The model under review builds one solid part; all positions refer to its coordinate system, in mm. Give positions to 0.01 mm unless a question says otherwise; leave off trailing zeros. Put each result on its own line as item: value.
```python
from build123d import *

# Parameters (mm, degrees)
SKETCH_3_R      = 1.700000006
SKETCH_3_R_2    = 1.100000006
SKETCH_3_W      = 12.5
SKETCH_3_H      = 23.5
EXTRUDE_2_DEPTH = 2


with BuildPart() as part:
    # 草图3 → 凸台-拉伸2 (new body)
    with BuildSketch(Plane.XY):
        with BuildLine():
            Line((16.840804288, 56.117583031), (0.840804288, 56.117583031))
            ThreePointArc((0.840804288, 56.117583031), (-0.573409274, 55.531796593), (-1.159195712, 54.117583031))
            Line((-1.159195712, 54.117583031), (-1.159195712, -100.882416969))
            ThreePointArc((-1.159195712, -100.882416969), (8.840804288, -110.882416969), (18.840804288, -100.882416969))
            Line((18.840804288, -100.882416969), (18.840804288, 54.117583031))
            ThreePointArc((18.840804288, 54.117583031), (18.255017851, 55.531796593), (16.840804288, 56.117583031))
        make_face()
        with Locations((8.840804288, -107.982416969)):
            Circle(SKETCH_3_R, mode=Mode.SUBTRACT)
        with BuildLine():
            ThreePointArc((10.540804288, -93.782416969), (7.63872276, -94.984498497), (8.840804288, -92.082416969))
            ThreePointArc((8.840804288, -92.082416969), (10.042885816, -92.580335441), (10.540804288, -93.782416969))
        make_face(mode=Mode.SUBTRACT)
        with BuildLine():
            ThreePointArc((10.540804294, -46.401557681), (10.04288582, -47.603639213), (8.840804288, -48.101557686))
            ThreePointArc((8.840804288, -48.101557686), (7.638722756, -45.199476149), (10.540804294, -46.401557681))
        make_face(mode=Mode.SUBTRACT)
        with Locations((8.840804288, -39.301557681)):
            Circle(SKETCH_3_R, mode=Mode.SUBTRACT)
        with Locations((8.840804288, -32.201557681)):
            Circle(SKETCH_3_R, mode=Mode.SUBTRACT)
        with Locations((8.840804288, -100.882416969)):
            Circle(SKETCH_3_R, mode=Mode.SUBTRACT)
        with BuildLine():
            add(Edge.make_bspline(
                [(8.840804288, -68.07230608), (10.518584029, -67.9276906), (13.271622127, -65.4378125), (9.324741551, -63.725127446)],
                knots=[0.615915535, 0.615915535, 0.615915535, 0.615915535, 1, 1, 1, 1], degree=3))
            add(Edge.make_bspline(
                [(5.004317127, -62.675716717), (6.671990842, -63.522758583), (7.358746233, -65.159768504), (7.765991833, -67.969605562), (8.568188953, -68.095804038), (8.840804288, -68.07230608)],
                knots=[0.002348501, 0.002348501, 0.002348501, 0.002348501, 0.410926836, 0.553507274, 0.615915535, 0.615915535, 0.615915535, 0.615915535], degree=3))
            add(Edge.make_bspline(
                [(4.975444833, -62.661146677), (4.985052333, -62.666591164), (4.994678321, -62.671455775), (5.004317127, -62.675716717)],
                knots=[0.565822578, 0.565822578, 0.565822578, 0.565822578, 0.579602808, 0.579602808, 0.579602808, 0.579602808], degree=3))
            add(Edge.make_bspline(
                [(4.278018154, -60.704640985), (4.226627162, -61.157219039), (4.526861731, -62.258746315), (4.916709377, -62.627861804), (4.975444833, -62.661146677)],
                knots=[0, 0, 0, 0, 0.481577142, 0.565822578, 0.565822578, 0.565822578, 0.565822578], degree=3))
            add(Edge.make_bspline(
                [(4.278018154, -60.704640985), (4.226627162, -60.252062931), (4.526861731, -59.150535655), (4.916709377, -58.781420166), (4.975444833, -58.748135293)],
                knots=[0, 0, 0, 0, 0.481577142, 0.565822578, 0.565822578, 0.565822578, 0.565822578], degree=3))
            add(Edge.make_bspline(
                [(4.975444833, -58.748135293), (4.985052333, -58.742690806), (4.994678321, -58.737826195), (5.004317127, -58.733565253)],
                knots=[0.565822578, 0.565822578, 0.565822578, 0.565822578, 0.579602808, 0.579602808, 0.579602808, 0.579602808], degree=3))
            add(Edge.make_bspline(
                [(5.004317127, -58.733565253), (6.671990842, -57.886523387), (7.358746233, -56.249513466), (7.765991833, -53.439676408), (8.568188953, -53.313477932), (8.840804288, -53.33697589)],
                knots=[0.002348501, 0.002348501, 0.002348501, 0.002348501, 0.410926836, 0.553507274, 0.615915535, 0.615915535, 0.615915535, 0.615915535], degree=3))
            add(Edge.make_bspline(
                [(8.840804288, -53.33697589), (10.518584029, -53.481591371), (13.271622127, -55.97146947), (9.324741551, -57.684154524)],
                knots=[0.615915535, 0.615915535, 0.615915535, 0.615915535, 1, 1, 1, 1], degree=3))
            add(Edge.make_bspline(
                [(9.324741551, -57.684154524), (9.448361201, -57.741607127), (9.579397012, -57.825403241)],
                knots=[0.879374293, 0.879374293, 0.879374293, 1, 1, 1], degree=2))
            add(Edge.make_bspline(
                [(9.579397012, -57.825403241), (10.442809677, -57.472287252), (11.335132803, -57.233463092), (12.256366661, -57.108930725)],
                knots=[0, 0, 0, 0, 0.985819408, 0.985819408, 0.985819408, 0.985819408], degree=3))
            add(Edge.make_bspline(
                [(12.256366661, -57.108930725), (12.250375457, -57.017628974), (12.324042897, -56.451578095), (14.134987008, -56.284356721), (14.027647091, -57.656331575), (13.69790824, -57.940504606)],
                knots=[0.192175897, 0.192175897, 0.192175897, 0.192175897, 0.262471761, 0.642903714, 1, 1, 1, 1], degree=3))
            add(Edge.make_bspline(
                [(13.69790824, -57.940504606), (14.014754559, -59.307854638), (13.928049408, -60.704640985)],
                knots=[0, 0, 0, 1, 1, 1], degree=2))
            add(Edge.make_bspline(
                [(13.69790824, -63.468777364), (14.014754559, -62.101427332), (13.928049408, -60.704640985)],
                knots=[0, 0, 0, 1, 1, 1], degree=2))
            add(Edge.make_bspline(
                [(12.256366661, -64.300351246), (12.250375457, -64.391652996), (12.324042897, -64.957703875), (14.134987008, -65.124925249), (14.027647091, -63.752950395), (13.69790824, -63.468777364)],
                knots=[0.192175897, 0.192175897, 0.192175897, 0.192175897, 0.262471761, 0.642903714, 1, 1, 1, 1], degree=3))
            add(Edge.make_bspline(
                [(9.579397012, -63.583878729), (10.442809677, -63.936994718), (11.335132803, -64.175818878), (12.256366661, -64.300351246)],
                knots=[0, 0, 0, 0, 0.985819408, 0.985819408, 0.985819408, 0.985819408], degree=3))
            add(Edge.make_bspline(
                [(9.324741551, -63.725127446), (9.448361201, -63.667674843), (9.579397012, -63.583878729)],
                knots=[0.879374293, 0.879374293, 0.879374293, 1, 1, 1], degree=2))
        make_face(mode=Mode.SUBTRACT)
        with Locations((8.840804288, -25.101557681)):
            Circle(SKETCH_3_R, mode=Mode.SUBTRACT)
        with Locations((8.840804288, -18.001557681)):
            Circle(SKETCH_3_R, mode=Mode.SUBTRACT)
        with Locations((8.840804288, -10.901557681)):
            Circle(SKETCH_3_R, mode=Mode.SUBTRACT)
        with Locations((8.840804288, -3.801557681)):
            Circle(SKETCH_3_R, mode=Mode.SUBTRACT)
        with Locations((8.840804288, 3.298442319)):
            Circle(SKETCH_3_R, mode=Mode.SUBTRACT)
        with Locations((2.140804288, 52.617583031)):
            Circle(SKETCH_3_R, mode=Mode.SUBTRACT)
        with Locations((8.840804288, 16.888295099)):
            Circle(SKETCH_3_R_2, mode=Mode.SUBTRACT)
        with Locations((8.840804288, 30.788295099)):
            Rectangle(SKETCH_3_W, SKETCH_3_H, mode=Mode.SUBTRACT)
        with Locations((8.840804288, 44.688295099)):
            Circle(SKETCH_3_R_2, mode=Mode.SUBTRACT)
        with Locations((15.540804288, 52.617583031)):
            Circle(SKETCH_3_R, mode=Mode.SUBTRACT)
    extrude(amount=EXTRUDE_2_DEPTH)


solid = part.part
```
(1) The part is to be moulded in two halves that separate along X. For faces 1 (the flat face through (6, -26, 0)), 2 (the cylindrical face through (8.62, -110.88, 0.99)), 3 (the cylindrical face through (8.47, -33.86, 0.99)), say which applies: pulls with the +X half, pulls with the -X half, needs draft (parallel to the pull), parting line crosses it, or undercut.
The answers:
face 1: needs draft
face 2: parting line crosses it
face 3: undercut
(2) Clearance check with a flat-ended pin moving along its axis: pin 1 Ø1.3 at (x, y) = (8.84, 16.89) entering from +Z. State where the tip first meets the part, or that it passes through.
The answers:
pin 1: through
(3) Take a section at A-A, the plane z = 1.3. Count the separate pieces of the cut face and the enclosed holes in it, then the cut area to 3 significant figures.
The answers:
separate pieces: 1
enclosed holes: 17
area: 2,790 mm^2
(4) Wall thickness on L1, parallel to Y at x = 14.25, z = 0.1; L2, parallel to X at y = 39, z = 0.4; L3, parallel to Y at x = 6, z = 1.7: over which ranges is each line inside the solid? List them lowest first.
The answers:
L1: -109.29 to 19.04, 42.54 to 51.51, 53.72 to 56.12
L2: -1.16 to 2.59, 15.09 to 18.84
L3: -110.47 to -63.33, -58.07 to 19.04, 42.54 to 56.12
